Could you check a few things on this model? Use its own coordinates, in mm. A direction names the side the tool comes from. Give positions to 0.01 mm unless a question says otherwise; leave off trailing zeros. Write each loop counter-clockwise with the first axis right and the second up, starting at its lowest first coordinate (ties: lowest second). Pieces come first, ordered by that corner, then holes. Notation, with made-up numbers: M -24.75,51 L 10.25,51 A21 cw 10.25,76 Z; hole C 4.25,76.5 d9. An arc over 180 degrees is marked long. One line per item, written item: value.
```python
from build123d import *

# Parameters (mm, degrees)
BOSS_EXTRUDE1_DEPTH = 4.65
SKETCH2_W           = 32
SKETCH2_H           = 19
CUT_EXTRUDE1_DEPTH  = 2.35
SKETCH3_W           = 7.5
SKETCH3_H           = 9.2
CUT_EXTRUDE2_DEPTH  = 2
SKETCH4_W           = 31
SKETCH4_H           = 45
CUT_EXTRUDE3_DEPTH  = 4.5
SKETCH5_W           = 53
SKETCH5_H           = 21.5
CUT_EXTRUDE4_DEPTH  = 4
CUT_EXTRUDE5_DEPTH  = 1.5
SKETCH7_W           = 25
SKETCH7_H           = 13.967841501
CUT_EXTRUDE6_DEPTH  = 1
SKETCH9_W           = 31.5
SKETCH9_H           = 70
CUT_EXTRUDE8_DEPTH  = 4


with BuildPart() as part:
    # Sketch1 → Boss-Extrude1 (new body)
    with BuildSketch(Plane(origin=(0, 0, 0), x_dir=(1, 0, 0), z_dir=(0, 1, 0))):
        with BuildLine():
            Line((0, 0), (211, 0))
            Line((211, 0), (211, 132))
            ThreePointArc((211, 132), (208.071067812, 139.071067812), (201, 142))
            Line((201, 142), (10, 142))
            ThreePointArc((10, 142), (2.928932188, 139.071067812), (0, 132))
            Line((0, 132), (0, 0))
        make_face()
    extrude(amount=BOSS_EXTRUDE1_DEPTH)

    # Sketch2 → Cut-Extrude1 (cut)
    with BuildSketch(Plane(origin=(0, 4.65, 0), x_dir=(1, 0, 0), z_dir=(0, 1, 0))):
        with Locations((16, 71)):
            Rectangle(SKETCH2_W, SKETCH2_H)
    extrude(amount=-CUT_EXTRUDE1_DEPTH, mode=Mode.SUBTRACT)

    # Sketch3 → Cut-Extrude2 (cut)
    with BuildSketch(Plane(origin=(0, 2.3, 0), x_dir=(1, 0, 0), z_dir=(0, 1, 0))):
        with Locations((3.75, 71)):
            Rectangle(SKETCH3_W, SKETCH3_H)
    extrude(amount=-CUT_EXTRUDE2_DEPTH, mode=Mode.SUBTRACT)

    # Sketch4 → Cut-Extrude3 (cut)
    with BuildSketch(Plane(origin=(0, 4.65, 0), x_dir=(1, 0, 0), z_dir=(0, 1, 0))):
        with Locations((73.681319495, 110.218338853)):
            Rectangle(SKETCH4_W, SKETCH4_H)
    extrude(amount=-CUT_EXTRUDE3_DEPTH, mode=Mode.SUBTRACT)

    # Sketch5 → Cut-Extrude4 (cut)
    with BuildSketch(Plane(origin=(0, 4.65, 0), x_dir=(1, 0, 0), z_dir=(0, 1, 0))):
        with Locations((139.927272952, 107.871903627)):
            Rectangle(SKETCH5_W, SKETCH5_H)
    extrude(amount=-CUT_EXTRUDE4_DEPTH, mode=Mode.SUBTRACT)

    # Sketch6 → Cut-Extrude5 (cut)
    with BuildSketch(Plane(origin=(0, 4.65, 0), x_dir=(1, 0, 0), z_dir=(0, 1, 0))):
        Polygon((32, 61.5), (79.5, 61.5), (79.5, 7.136151196), (131.5, 7.136151196), (131.5, 61.5), (182.227109874, 61.5), (182.261915258, 80.5), (177.949598934, 80.5), (177.678969488, 132.72), (92.678969488, 132.72), (92.678969488, 87.718338853), (89.181319495, 87.718338853), (89.181319495, 132.718338853), (58.181319495, 132.718338853), (58.181319495, 80.5), (32, 80.5), align=None)
    extrude(amount=-CUT_EXTRUDE5_DEPTH, mode=Mode.SUBTRACT)

    # Sketch7 → Cut-Extrude6 (cut)
    with BuildSketch(Plane(origin=(0, 4.65, 0), x_dir=(1, 0, 0), z_dir=(0, 1, 0))):
        with Locations((105.5, 6.983920751)):
            Rectangle(SKETCH7_W, SKETCH7_H)
    extrude(amount=-CUT_EXTRUDE6_DEPTH, mode=Mode.SUBTRACT)

    # Sketch9 → Cut-Extrude8 (cut)
    with BuildSketch(Plane(origin=(0, 4.65, 0), x_dir=(1, 0, 0), z_dir=(0, 1, 0))):
        with Locations((105.5, 44.997499802)):
            Rectangle(SKETCH9_W, SKETCH9_H)
    extrude(amount=-CUT_EXTRUDE8_DEPTH, mode=Mode.SUBTRACT)


solid = part.part
```
1) Please list where these lines run through material, in increasing order: L1, parallel to X at y = 0.8, z = -108.5; L2, parallel to X at y = 3.85, z = -38; L3, parallel to Z at x = 55, y = 3.85. Write a range as from..to.
Outcome:
L1: x = 0..58.18, 89.18..113.43, 166.43..211
L2: x = 0..79.5, 131.5..211
L3: z = -142..-80.5, -61.5..0
2) If we section it at C-C, the plane x = 53.5: Write out the boundary of the cut face in (y, z), then the cut area to 3 significant figures.
Outcome:
outline: M 0,-142 L 4.65,-142 L 4.65,-80.5 L 3.15,-80.5 L 3.15,-61.5 L 4.65,-61.5 L 4.65,0 L 0,0 Z
area: 632 mm^2
3) If we section it at A-A, the plane z = -29.5: Write out the boundary of the cut face in (x, y).
Outcome:
outline: M 0,0 L 211,0 L 211,4.65 L 131.5,4.65 L 131.5,3.15 L 121.25,3.15 L 121.25,0.65 L 89.75,0.65 L 89.75,3.15 L 79.5,3.15 L 79.5,4.65 L 0,4.65 Z
4) I'm going to push flat-ended pins straight in: pin 1 (0.6 mm diameter, centred on y = 1.5, z = -72.5, fed in from -X); pin 2 (3 mm diameter, centred on x = 72, z = -51, fed in from -Y); pin 3 (1 mm diameter, centred on x = 5, y = 1.5, fed in from -Z); pin 4 (6 mm diameter, centred on x = 5.5, z = -72, fed in from +Y). Where does each tip first touch, or does it pass through?
Outcome:
pin 1: stops at x = 7.5
pin 2: stops at y = 0
pin 3: stops at z = -140.93
pin 4: stops at y = 2.3
5) We'd pull the mould along X, two halves only. Please class faces 4 (the face through (104, 2, 0)), 5 (the face through (73, 2, -132.718)), 6 (the face through (3.01, 2.29, -139.15)), 7 (the face through (211, 2, -65)): pulls with the +X half, pulls with the -X half, needs draft (parallel to the pull), parting line crosses it, or undercut.
Outcome:
face 4: needs draft
face 5: undercut
face 6: pulls with the -X half
face 7: pulls with the +X half
6) If we section it at B-B, the plane x = 84: Write out the boundary of the cut face in (y, z), then the cut area to 3 significant figures.
Outcome:
outline: M 0,-142 L 4.65,-142 L 4.65,-132.72 L 0.15,-132.72 L 0.15,-87.72 L 3.15,-87.72 L 3.15,-7.14 L 4.65,-7.14 L 4.65,0 L 0,0 Z
area: 337 mm^2
7) If we section it at D-D, the plane z = -109: Write out the boundary of the cut face in (x, y), then the cut area to 3 significant figures.
Outcome:
outline: M 0,0 L 211,0 L 211,4.65 L 177.8,4.65 L 177.8,3.15 L 166.43,3.15 L 166.43,0.65 L 113.43,0.65 L 113.43,3.15 L 92.68,3.15 L 92.68,4.65 L 89.18,4.65 L 89.18,0.15 L 58.18,0.15 L 58.18,4.65 L 0,4.65 Z
area: 581 mm^2
8) On a 3-axis mill with a long thin cutter (end or side, diameter ignored), from which of +Z, -Z, +X, -X, +Y, -Y can I reach the whole of each face in a straight line? I mean faces 1 (the face through (105, 3.65, -4)), 2 (the face through (89.181, 2, -110)), 3 (the face through (4, 0.3, -71)). Say none if no direction works.
Outcome:
face 1: +Z, +Y
face 2: +Y
face 3: -X, +Y
